Autodesk Inventor part; units mm, degrees
ref_plane "YZ Plane" through (0, 0, 0) normal (1, 0, 0) x (0, 1, 0)
ref_plane "XZ Plane" through (0, 0, 0) normal (0, 1, 0) x (-1, 0, 0)
ref_plane "XY Plane" through (0, 0, 0) normal (0, 0, 1) x (1, 0, 0)
sketch "スケッチ1" plane through (0, 0, 0) normal (0, 1, 0) x (-1, 0, 0)
  line L0 (0, 0) -> (-5, 0)
  line L1 (-5, 0) -> (-5, -40)
  line L2 (-5, -40) -> (0, -40)
  line L3 (0, -40) -> (0, 0)
  dimension "d0" = 40
  dimension "d3" = 5
extrude "押し出し1" add sketch "スケッチ1" along normal blind 190
sketch "スケッチ2" plane through (5, 0, 0) normal (1, 0, 0) x (0, 0, -1)
  line L0 (0, 0) -> (0, 190)
  line L1 (0, 190) -> (40, 190)
  line L2 (0, 0) -> (0, 190)
  line L3 (40, 0) -> (40, 190)
  line L4 (0, 95) -> (40, 95)
  point P0 (4, 162.5)
  point P1 (28, 162.5)
  point P2 (4, 142.5)
  point P3 (28, 142.5)
  dimension "d4" = 4
  dimension "d5" = 27.5
  dimension "d8" = 24
  dimension "d11" = 20
hole "穴1" at (5, 162.5, -4) at (5, 162.5, -28) at (5, 142.5, -4) at (5, 142.5, -28) direction (-1, 0, 0) diameter 3.5 end through all
properties part number "縦フラットバー" material "アルミニウム"
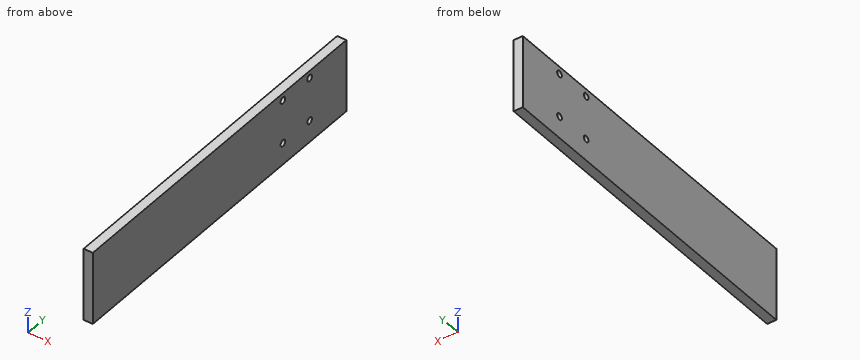
Design review of the part built by this model. Coordinates are the model's own, in mm. Give positions to 0.01 mm unless a question says otherwise; leave off trailing zeros. Loops run counter-clockwise (first coordinate to the right, second up) from the corner with the lowest first, then second, coordinate; pieces in that order, holes last. Notation, with made-up numbers: (-24.75, -19.5) - (-2.75, -19.5) arc R26 cw to (-2.75, 11.5) - close; hole circle Ø9 at (39.25, 81). An arc over 180 degrees is marked (long way). Write item = value, one per line.
1) Take a section at B-B on z = -4. State the section outline as (x, y) points.
Result sheet:
outline = (0, 0) - (5, 0) - (5, 140.75) - (0, 140.75) - close; (0, 144.25) - (5, 144.25) - (5, 160.75) - (0, 160.75) - close; (0, 164.25) - (5, 164.25) - (5, 190) - (0, 190) - close
2) To check wall thickness, follow line 1 (Y direction, x = 1.9, z = -4); line 2 (Z direction, x = 2.2, y = 162.5); line 3 (Z direction, x = 2.15, y = 143.5). State the ranges of each line that lie inside material, in increasing order.
Result sheet:
line_1 = 0 to 140.75, 144.25 to 160.75, 164.25 to 190
line_2 = -40 to -29.75, -26.25 to -5.75, -2.25 to 0
line_3 = -40 to -29.44, -26.56 to -5.44, -2.56 to 0
3) Clearance check with a flat-ended pin moving along its axis: pin 1 Ø5.5 at (y, z) = (142.5, -28) entering from -X. State where the tip first meets the part, or that it passes through.
Result sheet:
pin_1 = 0
4) Take a section at A-A on y = 162.5. State the section outline as (x, z) points.
Result sheet:
outline = (0, -40) - (5, -40) - (5, -29.75) - (0, -29.75) - close; (0, -26.25) - (5, -26.25) - (5, -5.75) - (0, -5.75) - close; (0, -2.25) - (5, -2.25) - (5, 0) - (0, 0) - close
